Check sheet for the modelled part. Datum: model origin and axes. Units: mm. A direction names the side the tool comes from. Coordinates: 2 decimals unless noted, no trailing zeros. Loops run counter-clockwise (first coordinate to the right, second up) from the corner with the lowest first, then second, coordinate; pieces in that order, holes last. Notation, with made-up numbers: M 57.5,31 L 114.5,31 A18 ccw 114.5,62 Z; hole C 57.25,76 d6. An arc over 180 degrees is marked long. Return JSON: item names as keys, results as strings.
from build123d import *

# Parameters (mm, degrees)
SKETCH1_R           = 5
BOSS_EXTRUDE1_DEPTH = 5
BOSS_EXTRUDE2_DEPTH = 2.5


with BuildPart() as part:
    # Sketch1 → Boss-Extrude1 (new, symmetric)
    with BuildSketch(Plane.XY):
        with BuildLine():
            Line((0, 16), (36.66060556, 16))
            ThreePointArc((36.66060556, 16), (4.629288395, 39.731218065), (-32, 24))
            ThreePointArc((-32, 24), (-35.527864045, 21.05572809), (-40, 20))
            Line((-40, 20), (-174.641016151, 20))
            ThreePointArc((-174.641016151, 20), (-194.641016151, 0), (-174.641016151, -20))
            Line((-174.641016151, -20), (-40, -20))
            ThreePointArc((-40, -20), (-35.527864045, -21.05572809), (-32, -24))
            ThreePointArc((-32, -24), (4.629288395, -39.731218065), (36.66060556, -16))
            Line((36.66060556, -16), (0, -16))
            ThreePointArc((0, -16), (-16, 0), (0, 16))
        make_face()
        with Locations((0, 28)):
            Circle(SKETCH1_R, mode=Mode.SUBTRACT)
        with Locations((0, -27)):
            Circle(SKETCH1_R, mode=Mode.SUBTRACT)
        with Locations((-28, 0)):
            Circle(SKETCH1_R, mode=Mode.SUBTRACT)
        with BuildLine():
            Line((-154.641016151, 8), (-54.641016151, 8))
            ThreePointArc((-54.641016151, 8), (-46.641016151, 0), (-54.641016151, -8))
            Line((-54.641016151, -8), (-154.641016151, -8))
            ThreePointArc((-154.641016151, -8), (-162.641016151, 0), (-154.641016151, 8))
        make_face(mode=Mode.SUBTRACT)
    extrude(amount=BOSS_EXTRUDE1_DEPTH, both=True)

    # Sketch1<2> → Boss-Extrude2 (add, symmetric)
    with BuildSketch(Plane.XY):
        with BuildLine():
            Line((-154.641016151, -8), (-54.641016151, -8))
            ThreePointArc((-54.641016151, -8), (-46.641016151, 0), (-54.641016151, 8))
            Line((-54.641016151, 8), (-154.641016151, 8))
            ThreePointArc((-154.641016151, 8), (-162.641016151, 0), (-154.641016151, -8))
        make_face()
    extrude(amount=BOSS_EXTRUDE2_DEPTH, both=True)


solid = part.part
1) Scan lines: line 1 along Y through (x, z) = (0, 3); line 2 along Y through (x, z) = (-126, 2.75); line 3 along Z through (x, y) = (-123, 4.5). Record each from-to range of solid material in increasing order. Write a range as [from, to].
Answers:
{"line 1": "[-40, -32], [-22, -16], [16, 23], [33, 40]", "line 2": "[-20, -8], [8, 20]", "line 3": "[-2.5, 2.5]"}
2) Draft check along Y on faces 6 (the face through (-1.08, -31.88, -0.07)), 7 (the face through (-108, -20, 0)), 8 (the face through (-35.47, 21.085, 0.07)). Enter one of: +Y half, -Y half, draft (parallel to the pull), parting line (faces both ways), or undercut.
Answers:
{"face 6": "undercut", "face 7": "-Y half", "face 8": "+Y half"}
3) Section check A-A on z = 0. Record the cut outline in (x, y).
Answers:
{"outline": "M -174.64,-20 L -40,-20 A10 cw -32,-24 A40 ccw 36.66,-16 L 0,-16 A16 cw 0,16 L 36.66,16 A40 ccw -32,24 A10 cw -40,20 L -174.64,20 A20 ccw Z; hole C -28,0 d10; hole C 0,-27 d10; hole C 0,28 d10"}
4) Section check B-B on x = -28. Record the cut outline in (y, z).
Answers:
{"outline": "M -28.57,-5 L -5,-5 L -5,5 L -28.57,5 Z; M 5,-5 L 28.57,-5 L 28.57,5 L 5,5 Z"}
5) Section check D-D on x = -61. Record the cut outline in (y, z).
Answers:
{"outline": "M -20,-5 L -8,-5 L -8,-2.5 L 8,-2.5 L 8,-5 L 20,-5 L 20,5 L 8,5 L 8,2.5 L -8,2.5 L -8,5 L -20,5 Z"}
6) Go/stop test with flat-tipped pins: pin 1 Ø5 at (x, y) = (-126.5, -1) entering from -Z; pin 2 Ø2 at (x, z) = (-87.5, 4.5) entering from +Y; pin 3 Ø17.5 at (x, y) = (-125, -3.5) entering from +Z; pin 4 Ø5 at (x, z) = (14, -1) entering from +Y. Record where each tip stops, or that it passes through.
Answers:
{"pin 1": "z = -2.5", "pin 2": "y = 20", "pin 3": "z = 5", "pin 4": "y = 38.31"}
7) Set-up check for faces 1 (the face through (-105, 0, 2.5)), 2 (the face through (-46.643, 0.176, -3.732)), 3 (the face through (19, -16, 0)), 4 (the face through (-106, 20, 0)), 5 (the face through (5.21, 39.66, 0.07)): record each of +Z, -Z, +X, -X, +Y, -Y from which the full face is reachable in a straight line by a thin tool's end or side.
Answers:
{"face 1": "+Z", "face 2": "-Z", "face 3": "+Z, -Z, +X", "face 4": "+Z, -Z, -X, +Y", "face 5": "+Z, -Z, +Y"}
